```python
from build123d import *

# Parameters (mm, degrees)
PAD_DEPTH        = 3
SKETCH001_R      = 1.7
POCKET_DEPTH     = 3
SKETCH002_W      = 13
SKETCH002_H      = 3
PAD001_DEPTH     = 10
PAD002_DEPTH     = 10
SKETCH011_R      = 2.3
POCKET003_DEPTH  = 3
POCKET004_DEPTH  = 4
HOLE_D           = 1.75
HOLE_DEPTH       = 25
HOLE_CSINK_D     = 7
HOLE_CSINK_ANGLE = 90


with BuildPart() as part:
    # Sketch → Pad (new body)
    with BuildSketch(Plane.XY):
        Polygon((-17, 26.5), (27.5, 26.5), (27.499024, -5.5), (-17.001501, -5.5), align=None)
    extrude(amount=PAD_DEPTH)

    # Sketch001 (on Face6 of Pad) → Pocket (cut)
    with BuildSketch(Plane.XY.offset(3)):
        with Locations((-7, 22)):
            Circle(SKETCH001_R)
        with Locations((-7, 14)):
            Circle(SKETCH001_R)
        with Locations((6, 16)):
            Circle(SKETCH001_R)
        with Locations((21, 16)):
            Circle(SKETCH001_R)
        with Locations((6, 5.864343)):
            Circle(SKETCH001_R)
        with Locations((20.999966, 5.832606)):
            Circle(SKETCH001_R)
    extrude(amount=-POCKET_DEPTH, mode=Mode.SUBTRACT)

    # Sketch002 (on Face2 of Pocket) → Pad001 (join)
    with BuildSketch(Plane(origin=(-17.001243, 0.000797, 0), x_dir=(-4.7e-05, -1, 0), z_dir=(-1, 4.7e-05, 0))):
        with Locations((-11.5, 1.5)):
            Rectangle(SKETCH002_W, SKETCH002_H)
    extrude(amount=PAD001_DEPTH)

    # Sketch003 (on Face3 of Pad001) → Pad002 (join)
    with BuildSketch(Plane(origin=(27.499192, -0.000839, 0), x_dir=(3e-05, 1, 0), z_dir=(1, -3e-05, 0))):
        Polygon((5, -5.3e-05), (18, 0.009854), (18, 3.010224), (5, 3.000316), align=None)
    extrude(amount=PAD002_DEPTH)

    # Sketch011 (on Face10 of Pad002) → Pocket003 (cut)
    with BuildSketch(Plane(origin=(0, 0, 0), x_dir=(1, 0, 0), z_dir=(0, 0, -1))):
        with Locations((-21.745842, -11)):
            Circle(SKETCH011_R)
        with Locations((29.89052, -11)):
            Circle(SKETCH011_R)
    extrude(amount=-POCKET003_DEPTH, mode=Mode.SUBTRACT)

    # Sketch011 (on Face10 of Pad002) → Pocket004 (cut)
    with BuildSketch(Plane(origin=(0, 0, 0), x_dir=(1, 0, 0), z_dir=(0, 0, -1))):
        with Locations((-21.745842, -11)):
            Circle(SKETCH011_R)
        with Locations((29.89052, -11)):
            Circle(SKETCH011_R)
    extrude(amount=-POCKET004_DEPTH, mode=Mode.SUBTRACT)

    # Hole
    with Locations(Plane.XY.offset(3)):
        with Locations((-7, 22), (-7, 14), (6, 16), (21, 16), (6, 5.864343), (20.999966, 5.832606)):
            CounterSinkHole(HOLE_D / 2, HOLE_CSINK_D / 2, depth=HOLE_DEPTH, counter_sink_angle=HOLE_CSINK_ANGLE)


solid = part.part
```
Can you work these out from the model? Positions are in its coordinate system, mm. Coordinates: 2 decimals unless noted, no trailing zeros. Write each loop counter-clockwise with the first axis right and the second up, starting at its lowest first coordinate (ties: lowest second). Pieces come first, ordered by that corner, then holes. Notation, with made-up numbers: M 34.25,47.5 L 52.25,47.5 A12 cw 52.25,52.5 Z; hole C 31,8.5 d2. An arc over 180 degrees is marked long. Write item = value, one per line. Start each with the question number.
Q1. I'm going to push flat-ended pins straight in: pin 1 (2 mm diameter, centred on x = 14.5, y = 3.5, fed in from +Z); pin 2 (0.9 mm diameter, centred on y = 22, z = 2, fed in from -X); pin 3 (1.5 mm diameter, centred on x = -24, z = 1, fed in from -Y). Where does each tip first touch, or does it pass through?
Q2. If we section it at C-C, the plane x = 29: Write out the boundary of the cut face in (y, z).
Q3. Thinking about a two-plate mould opening in X: for faces 1 (the face through (-20.51, 9.06, 1.48)), 2 (the face through (1, 11, 3)), which applies, released by +X, released by -X, zero draft, split by the parting line, or undercut?
Q4. If we section it at B-B, the plane z = 1.7: State how many separate pieces and enclosed holes the cut face has, then the cut area to 3 significant figures.
Q5. If we section it at A-A, the plane x = -7: Write out the boundary of the cut face in (y, z).
Q6. If I drill on L1, parallel to X at y = 16, z = 0.85; L2, parallel to Y at x = -7, z = 0.45; L3, parallel to Y at x = 6, z = 0.35, over which ranges is the centre line in solid material (lowest first)? Write a range as [from, to].
Q7. If we section it at D-D, the plane y = -2: Write out the boundary of the cut face in (x, z), then the cut area to 3 significant figures.
Check sheet entries:
q1.pin_1 = 3
q1.pin_2 = -17
q1.pin_3 = 5
q2.outline = M 5,0 L 8.88,0 L 8.88,3 L 5,3 Z; M 13.12,0.01 L 18,0.01 L 18,3.01 L 13.12,3.01 Z
q3.face_1 = undercut
q3.face_2 = zero draft
q4.separate_pieces = 1
q4.enclosed_holes = 8
q4.area = 1,560 mm²
q5.outline = M -5.5,0 L 12.3,0 L 12.3,1.2 L 10.5,3 L -5.5,3 Z; M 15.7,0 L 20.3,0 L 20.3,1.2 L 18.5,3 L 17.5,3 L 15.7,1.2 Z; M 23.7,0 L 26.5,0 L 26.5,3 L 25.5,3 L 23.7,1.2 Z
q6.L1 = [-27, 4.3], [7.7, 19.3], [22.7, 37.5]
q6.L2 = [-5.5, 12.3], [15.7, 20.3], [23.7, 26.5]
q6.L3 = [-5.5, 4.16], [7.56, 14.3], [17.7, 26.5]
q7.outline = M -17,0 L 27.5,0 L 27.5,3 L -17,3 Z
q7.area = 134 mm²
